```python
from build123d import *

# Parameters (mm, degrees)
SKETCH3_R           = 17.5
SKETCH3_R_2         = 1.25
SKETCH3_R_3         = 5.5
SKETCH3_R_4         = 2
BOSS_EXTRUDE2_DEPTH = 36
BOSS_EXTRUDE3_START = 36
SKETCH3_4_R         = 2
BOSS_EXTRUDE3_DEPTH = 16
BOSS_EXTRUDE4_START = -2
SKETCH3_5_R         = 5.5
SKETCH3_5_R_2       = 2
BOSS_EXTRUDE4_DEPTH = 2
SKETCH3_8_R         = 1.25
CUT_EXTRUDE1_DEPTH  = 3.5
CUT_EXTRUDE2_START  = 36
BASE_R              = 1.5
CUT_EXTRUDE2_DEPTH  = 3
BOSS_EXTRUDE5_START = 30
BOSS_EXTRUDE5_DEPTH = 4


with BuildPart() as part:
    # Sketch3 → Boss-Extrude2 (new body)
    # profile 1 of 6: a face of its own
    with BuildSketch(Plane.XY):
        Circle(SKETCH3_R)
        with Locations((-6.495190528, -3.75)):
            Circle(SKETCH3_R_2, mode=Mode.SUBTRACT)
        with Locations((6.495190528, -3.75)):
            Circle(SKETCH3_R_2, mode=Mode.SUBTRACT)
        with Locations((0, 7.5)):
            Circle(SKETCH3_R_2, mode=Mode.SUBTRACT)
        Circle(SKETCH3_R_3, mode=Mode.SUBTRACT)
    # profile 2 of 6: a face of its own
    with BuildSketch(Plane.XY):
        with Locations((0, 7.5)):
            Circle(SKETCH3_R_2)
    # profile 3 of 6: a face of its own
    with BuildSketch(Plane.XY):
        Circle(SKETCH3_R_3)
        Circle(SKETCH3_R_4, mode=Mode.SUBTRACT)
    # profile 4 of 6: a face of its own
    with BuildSketch(Plane.XY):
        Circle(SKETCH3_R_4)
    # profile 5 of 6: a face of its own
    with BuildSketch(Plane.XY):
        with Locations((-6.495190528, -3.75)):
            Circle(SKETCH3_R_2)
    # profile 6 of 6: a face of its own
    with BuildSketch(Plane.XY):
        with Locations((6.495190528, -3.75)):
            Circle(SKETCH3_R_2)
    extrude(amount=BOSS_EXTRUDE2_DEPTH)

    # Sketch3<4> → Boss-Extrude3 (add)
    with BuildSketch(Plane.XY.offset(BOSS_EXTRUDE3_START)):
        Circle(SKETCH3_4_R)
    extrude(amount=BOSS_EXTRUDE3_DEPTH)

    # Sketch3<5> → Boss-Extrude4 (add)
    with BuildSketch(Plane.XY.offset(BOSS_EXTRUDE4_START)):
        Circle(SKETCH3_5_R)
        Circle(SKETCH3_5_R_2, mode=Mode.SUBTRACT)
    extrude(amount=BOSS_EXTRUDE4_DEPTH)

    # Sketch3<8> → Cut-Extrude1 (cut)
    with BuildSketch(Plane.XY):
        with Locations((0, 7.5)):
            Circle(SKETCH3_8_R)
        with Locations((6.495190528, -3.75)):
            Circle(SKETCH3_8_R)
        with Locations((-6.495190528, -3.75)):
            Circle(SKETCH3_8_R)
    extrude(amount=CUT_EXTRUDE1_DEPTH, mode=Mode.SUBTRACT)

    # Base → Cut-Extrude2 (cut)
    with BuildSketch(Plane.XY.offset(CUT_EXTRUDE2_START)):
        with Locations((8.838834765, 8.838834765)):
            Circle(BASE_R)
        with Locations((-6.717514421, 6.717514421)):
            Circle(BASE_R)
        with Locations((-8.838834765, -8.838834765)):
            Circle(BASE_R)
        with Locations((6.717514421, -6.717514421)):
            Circle(BASE_R)
    extrude(amount=-CUT_EXTRUDE2_DEPTH, mode=Mode.SUBTRACT)

    # Base<4> → Boss-Extrude5 (add)
    with BuildSketch(Plane.XY.offset(BOSS_EXTRUDE5_START)):
        with BuildLine():
            ThreePointArc((-17.24093965, -3), (-17.5, 0), (-17.24093965, 3))
            Line((-17.24093965, 3), (-22.5, 2))
            Line((-22.5, 2), (-22.5, -2))
            Line((-22.5, -2), (-17.24093965, -3))
        make_face()
    extrude(amount=BOSS_EXTRUDE5_DEPTH)


solid = part.part
```
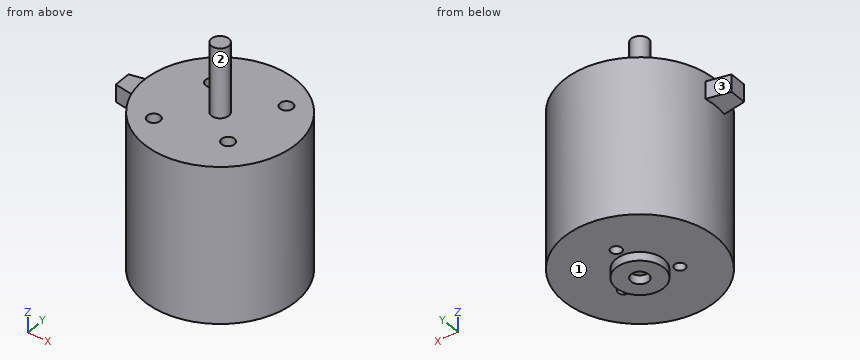
CAD build for the part. Positions are in the model's coordinates, mm. Face numbers are marked on the shaded views. A direction names the side the tool comes from. Coordinates: 2 decimals unless noted, no trailing zeros. Order: outer loops, then holes, each group sorted by start corner. A loop starts at its lowest first (then second) coordinate and runs counter-clockwise, first axis right, second up. Notation, with made-up numbers: (43.25, 51.5) - (96.25, 51.5) arc R24 ccw to (96.25, 80.5) - close; hole circle Ø7 at (73.5, 51). An arc over 180 degrees is marked (long way). Use a Markdown table: item, result. Add a question column.
(1) Flat gauge pins, fed straight in: pin 1 (1.2 mm diameter, centred on x = 0, y = 7, fed in from -Z); pin 2 (1.8 mm diameter, centred on x = -6.72, y = 6.72, fed in from +Z); pin 3 (10 mm diameter, centred on x = -4.5, y = 9, fed in from +Z). Where does each tip first touch, or does it go through?
(2) Saw through at D-D (z = 41). Give the cut face in (x, y), then the cut area to 3 significant figures.
(3) Drill centre lines: line 1 along Y through (x, z) = (0, -0.9); line 2 along Z through (x, y) = (9.5, 14); line 3 along Y through (x, z) = (7, 1). Where is each one in solid material? Low to high. Write a range as [from, to].
(4) Saw through at C-C (z = 22). Give the cut face in (x, y), then the cut area to 3 significant figures.
(5) Which spindle directions (+Z, -Z, +X, -X, +Y, -Y) get a long thin tool onto all of the face, cutting with end or side? Do the marked faces 1, 2 and 3. Say none if no direction does.
(6) Saw through at B-B (y = 0). Give the cut face in (x, z).
(7) Saw through at A-A (x = 0). Give the cut face in (y, z), then the cut area to 3 significant figures.
Solved:
| question | item | result |
|---|---|---|
| 1 | pin 1 | stops at z = 3.5 |
| 1 | pin 2 | stops at z = 33 |
| 1 | pin 3 | stops at z = 36 |
| 2 | outline | circle Ø4 at (0, 0) |
| 2 | area | 12.6 mm² |
| 3 | line 1 | y = [-5.5, -2], [2, 5.5] |
| 3 | line 2 | z = [0, 36] |
| 3 | line 3 | y = [-16.04, -4.89], [-2.61, 16.04] |
| 4 | outline | circle Ø35 at (0, 0) |
| 4 | area | 962 mm² |
| 5 | face 1 | -Z |
| 5 | face 2 | +Z |
| 5 | face 3 | +Z, -Z, -X, +Y |
| 6 | outline | (-22.5, 30) - (-17.5, 30) - (-17.5, 0) - (-5.5, 0) - (-5.5, -2) - (-2, -2) - (-2, 0) - (2, 0) - (2, -2) - (5.5, -2) - (5.5, 0) - (17.5, 0) - (17.5, 36) - (2, 36) - (2, 52) - (-2, 52) - (-2, 36) - (-17.5, 36) - (-17.5, 34) - (-22.5, 34) - close |
| 7 | outline | (-17.5, 0) - (-5.5, 0) - (-5.5, -2) - (-2, -2) - (-2, 0) - (2, 0) - (2, -2) - (5.5, -2) - (5.5, 0) - (6.25, 0) - (6.25, 3.5) - (8.75, 3.5) - (8.75, 0) - (17.5, 0) - (17.5, 36) - (2, 36) - (2, 52) - (-2, 52) - (-2, 36) - (-17.5, 36) - close |
| 7 | area | 1,330 mm² |
